Source: CAD feature listing. Evaluate the final solid. Frame: model axes, mm. Face numbers are marked on the shaded views. A direction names the side the tool comes from. Coordinates: 2 decimals unless noted, no trailing zeros. Loops run counter-clockwise (first coordinate to the right, second up) from the corner with the lowest first, then second, coordinate; pieces in that order, holes last. Notation, with made-up numbers: (15, 13.25) -> (67, 13.25) arc R21 ccw to (67, 21.25) -> close; hole circle Ø9 at (-0.75, 63.25). An arc over 180 degrees is marked (long way). Answer as CSV lines item,"result".
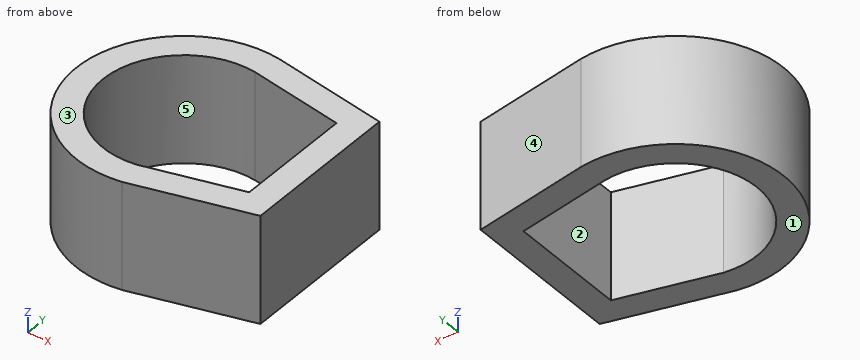
from build123d import *

# Parameters (mm, degrees)
SALIENTE_EXTRUIR1_DEPTH = 20


with BuildPart() as part:
    # Croquis3 → Saliente-Extruir1 (new body)
    with BuildSketch(Plane.XY):
        with BuildLine():
            Line((-4.157247249, 6.116640811), (-26.038869698, 10.382100053))
            ThreePointArc((-26.038869698, 10.382100053), (-49.345509053, -9.429582016), (-26.215773458, -29.447511872))
            Line((-26.215773458, -29.447511872), (-4.157247249, -24.2640649))
            Line((-4.157247249, -24.2640649), (-4.157247249, 6.116640811))
        make_face()
        with BuildLine():
            Line((-9.157247249, 1.997195972), (-26.902985069, 5.456433128))
            ThreePointArc((-26.902985069, 5.456433128), (-44.345215717, -9.396971545), (-27.144674573, -24.529599364))
            Line((-27.144674573, -24.529599364), (-9.157247249, -20.302804028))
            Line((-9.157247249, -20.302804028), (-9.157247249, 1.997195972))
        make_face(mode=Mode.SUBTRACT)
    extrude(amount=SALIENTE_EXTRUIR1_DEPTH)


solid = part.part
(1) Access query for the marked faces 1 and 2. Directions: +Z, -Z, +X, -X, +Y, -Y. A direction counts if a zero-diameter tool reaches every point of the face in a straight line with its end or side. Return the directions, or none.
Computed values:
face 1,"-Z, +X, -X, +Y, -Y"
face 2,"+Z, -Z"
(2) Draft query along X for the marked faces 3, 4 and 5. Return one class per face: released by +X, released by -X, zero draft, split by the parting line, or undercut.
Computed values:
face 3,"zero draft"
face 4,"released by +X"
face 5,"undercut"
(3) Cut plane A-A (y = -8). Return the cut outline in (x, z), then the cut area to 3 significant figures.
Computed values:
outline,"(-49.29, 0) -> (-44.27, 0) -> (-44.27, 20) -> (-49.29, 20) -> close; (-9.16, 0) -> (-4.16, 0) -> (-4.16, 20) -> (-9.16, 20) -> close"
area,"200 mm^2"
(4) Pin query (flat end, axial travel): pin 1 Ø1 at (x, y) = (-42, -15) entering from -Z; pin 2 Ø3 at (x, z) = (-31, 18) entering from -Y; pin 3 Ø6 at (x, z) = (-21.5, 12.5) entering from +Y. Return the tip coordinate at first contact, or that it passes through.
Computed values:
pin 1,"through"
pin 2,"y = -29.67"
pin 3,"y = 10.08"
(5) Cut plane D-D (x = -46). Return the cut outline in (y, z), then the cut area to 3 significant figures.
Computed values:
outline,"(-20.64, 0) -> (1.6, 0) -> (1.6, 20) -> (-20.64, 20) -> close"
area,"445 mm^2"
(6) Cut plane B-B (z = 3). Return the cut outline in (x, y), then the cut area to 3 significant figures.
Computed values:
outline,"(-26.22, -29.45) -> (-4.16, -24.26) -> (-4.16, 6.12) -> (-26.04, 10.38) arc R20.15 ccw (long way) to start; hole (-27.14, -24.53) -> (-9.16, -20.3) -> (-9.16, 2) -> (-26.9, 5.46) arc R15.15 ccw (long way) to start"
area,"639 mm^2"
(7) Cut plane C-C (x = -39). Return the cut outline in (y, z).
Computed values:
outline,"(-27.12, 0) -> (-21.07, 0) -> (-21.07, 20) -> (-27.12, 20) -> close; (2.03, 0) -> (8.08, 0) -> (8.08, 20) -> (2.03, 20) -> close"
(8) Material intervals for L1, parallel to X at y = -7.5, z = 9.75; L2, parallel to Y at x = -19, z = 6.5; L3, parallel to Y at x = -29.5, z = 1.75, sorted ascending. Write a range as [from, to].
Computed values:
L1,"[-49.24, -44.21], [-9.16, -4.16]"
L2,"[-27.75, -22.62], [3.92, 9.01]"
L3,"[-29.67, -24.67], [5.63, 10.63]"
